Geometry: final body of the model. Coordinates: model frame, mm. Give positions to 0.01 mm unless a question says otherwise; leave off trailing zeros. Write each loop counter-clockwise with the first axis right and the second up, starting at its lowest first coordinate (ties: lowest second). Pieces come first, ordered by that corner, then holes. Notation, with made-up numbers: (59.25, 35) -> (75.25, 35) arc R10 cw to (75.25, 48) -> close; hole circle Ø2 at (84, 57). An arc over 180 degrees is marked (long way). Answer as a JSON object with one key per item and string values. Group by question number.
(1) Section query D-D on x = -14.5. Output: boundary loops of the cut face in (y, z), plus the area to 3 significant figures.
(2) Section query C-C on y = 34. Output: boundary loops of the cut face in (x, z).
(3) Section query B-B on z = 2.1. State how many separate pieces and enclosed holes the cut face has, plus the area to 3 significant figures.
(4) Material intervals for probe 1 along X at (y, z) = (50.5, 0.8); probe 2 along X at (y, z) = (43, 0.5); probe 3 along Y at (x, z) = (-8.5, 0.2), sorted ascending.
(5) Draft query along Y for faces 1 (the face through (8.02, 59.215, 1.479)), 2 (the face through (-50.516, 22.142, 1.479)), 3 (the face through (-26.851, 41.377, 1.521)), 4 (the face through (8.1, 50.194, 1.479)). Return one class per face: +Y half, -Y half, draft (parallel to the pull), parting line (faces both ways), or undercut.
(6) Contact query for a flat-ended pin moving along its axis: pin 1 Ø4 at (x, y) = (-42.89, 18.39) entering from -Z. Output: stop coordinate, or through.
(7) Section query A-A on x = 6.5. Output: boundary loops of the cut face in (y, z).
Autodesk Inventor part; units mm, degrees
ref_plane "YZ Plane" through (0, 0, 0) normal (1, 0, 0) x (0, 1, 0)
ref_plane "XZ Plane" through (0, 0, 0) normal (0, 1, 0) x (-1, 0, 0)
ref_plane "XY Plane" through (0, 0, 0) normal (0, 0, 1) x (1, 0, 0)
sketch "スケッチ1" plane through (0, 0, 0) normal (0, 0, 1) x (1, 0, 0)
  circle A0 centre (0, 0) radius 20.55 construction
  circle A1 centre (-21.6908, -16.4118) radius 19.1 construction
  circle A2 centre (25.3202, -9.9362) radius 19.1 construction
  circle A3 centre (-50.601, 30.8143) radius 1.5
  circle A4 centre (5.9362, 53.5882) radius 1.5
  circle A5 centre (27.3908, 10.6821) radius 1.5
  circle A6 centre (-42.8914, 18.3887) radius 1.5
  circle A7 centre (-21.6908, -16.4118) radius 4.025
  circle A8 centre (25.3202, -9.9362) radius 4.025
  circle A9 centre (0, 0) radius 4
  line L0 (-17.8785, -18.8026) -> (-30.4168, -38.7963) construction
  arc A10 (-17.8785, -18.8026) -> (-19.2493, -12.6317) centre (-21.6908, -16.4118) ccw construction
  line L1 (-19.2493, -12.6317) -> (-39.0737, 0.1727) construction
  line L2 (37.1409, -30.8522) -> (21.8866, -12.8448) construction
  arc A11 (22.3659, -6.5417) -> (21.8866, -12.8448) centre (25.3202, -9.9362) ccw construction
  line L3 (22.3659, -6.5417) -> (40.1678, 8.9519) construction
  line L4 (-21.6908, -16.4118) -> (-99.9742, 13.5882) construction
  line L5 (-105.5257, -16.4118) -> (-21.6908, -16.4118) construction
  line L6 (-21.6908, -16.4118) -> (-101.7113, -41.4118) construction
  line L7 (25.3202, -9.9362) -> (102.5386, -46.4118) construction
  line L8 (110.4743, -16.4118) -> (25.3202, -9.9362) construction
  line L9 (25.3202, -9.9362) -> (108.6869, 8.5882) construction
  line L10 (-18.0583, -13.7557) -> (-31.9879, 5.2949) construction
  line L11 (-17.339, -17.5569) -> (-24.5367, -44.9106) construction
  line L12 (21.5077, -7.5456) -> (34.045, 12.4488) construction
  line L13 (21.0739, -11.4259) -> (31.6059, -41.446) construction
  arc A12 (-24.6176, -40.3201) -> (-19.5065, -44.4166) centre (-20.132, -39.9603) ccw
  circle A13 centre (-20.132, -39.9603) radius 3 construction
  arc A14 (-38.9879, 7.9907) -> (-39.3359, 8.5262) centre (-35.3982, 10.7044) ccw construction
  circle A15 centre (-35.3982, 10.7044) radius 3 construction
  arc A16 (-31.9879, 5.2949) -> (-33.8465, 6.7744) centre (-35.6204, 2.6388) ccw construction
  circle A17 centre (-41.5152, -3.6073) radius 1.5
  line L14 (-33.8465, 6.7744) -> (-56.066, 16.3055) construction
  line L15 (-41.3386, 0.8892) -> (-72.6317, 2.1181) construction
  circle A18 centre (-42.8914, 18.3887) radius 3 construction
  circle A19 centre (-35.3982, 10.7044) radius 1.5
  circle A20 centre (36.7736, 17.5344) radius 1.5
  arc A21 (40.7942, 15.5132) -> (40.1934, 20.4593) centre (36.7736, 17.5344) ccw
  circle A22 centre (25.6508, -33.5339) radius 1.5
  arc A23 (26.2763, -37.9902) -> (30.1508, -33.5178) centre (25.6508, -33.5339) ccw
  circle A24 centre (36.7736, 17.5344) radius 3 construction
  circle A25 centre (25.6508, -33.5339) radius 3 construction
  arc A26 (36.6836, 14.4025) -> (34.045, 12.4488) centre (37.8575, 10.0583) ccw construction
  line L16 (36.6836, 14.4025) -> (64.1968, 21.8369) construction
  line L17 (43.2599, 10.0553) -> (82.9273, 8.8396) construction
  circle A27 centre (27.3908, 10.6821) radius 3 construction
  circle A28 centre (-21.6908, -16.4118) radius 7.025 construction
  circle A29 centre (25.3202, -9.9362) radius 7.025 construction
  arc A30 (40.8593, 15.6483) -> (30.1508, -33.5178) centre (146.4685, -33.1029) ccw
  arc A31 (-24.6176, -40.3201) -> (-39.1827, 8.2484) centre (-145.1158, -49.988) ccw
  arc A32 (-52.2824, 34.9884) -> (-54.1907, 28.1005) centre (-50.601, 30.8143) ccw
  arc A33 (9.356, 56.5132) -> (4.2549, 57.7623) centre (5.9362, 53.5882) ccw
  line L18 (-39.1827, 8.2484) -> (-54.1907, 28.1005)
  line L19 (-52.2824, 34.9884) -> (4.2549, 57.7623)
  line L20 (9.356, 56.5132) -> (40.1934, 20.4593)
  line L21 (-19.5065, -44.4166) -> (26.2763, -37.9902)
  circle A34 centre (-20.132, -39.9603) radius 1.5
  line L22 (-23.8868, -42.4405) -> (-17.339, -17.5569)
  arc A35 (-17.339, -17.5569) -> (-18.0583, -13.7557) centre (-21.6908, -16.4118) ccw
  line L23 (-18.0583, -13.7557) -> (-31.9879, 5.2949)
  arc A36 (-31.9879, 5.2949) -> (-33.8465, 6.7744) centre (-35.6204, 2.6388) ccw
  line L24 (-33.8465, 6.7744) -> (-40.0946, 9.4545)
  line L25 (40.7974, 15.5141) -> (36.6836, 14.4025)
  arc A37 (36.6836, 14.4025) -> (34.045, 12.4488) centre (37.8575, 10.0583) ccw
  line L26 (34.045, 12.4488) -> (21.5077, -7.5456)
  arc A38 (21.5077, -7.5456) -> (21.0739, -11.4259) centre (25.3202, -9.9362) ccw
  line L27 (21.0739, -11.4259) -> (29.592, -35.7057)
  dimension "d0" = 8.05
  dimension "d1" = 8.05
  dimension "d2" = 8
  dimension "d3" = 20.968
  dimension "d4" = 20.968
  dimension "d5" = 17.35
  dimension "d6" = 17.35
  dimension "d7" = 16.877
  dimension "d8" = 16.877
  dimension "d9" = 20.936
  dimension "d10" = 20.936
  dimension "d11" = 9
  dimension "d12" = 6
  dimension "d13" = 9
  dimension "d14" = 6
  dimension "d15" = 9
  dimension "d16" = 20.968
  dimension "d17" = 20.968
  dimension "d18" = 6
  dimension "d19" = 3
  dimension "d20" = 3
  dimension "d21" = 9
  dimension "d22" = 3
  dimension "d23" = 9
  dimension "d24" = 6
  dimension "d25" = 6
  dimension "d26" = 9
  dimension "d27" = 16.877
  dimension "d28" = 3
  dimension "d29" = 3
  dimension "d30" = 9
  dimension "d31" = 9
  dimension "d32" = 3
sketch "スケッチ2" plane through (0, 0, 0) normal (0, 0, 1) x (1, 0, 0)
  circle A0 centre (-50.601, 30.8143) radius 1.5
  circle A1 centre (-42.8914, 18.3887) radius 1.5
  circle A2 centre (5.9362, 53.5882) radius 1.5
  circle A3 centre (27.3908, 10.6821) radius 1.5
  arc A4 (-52.3846, 34.9457) -> (-54.4248, 28.4418) centre (-50.601, 30.8143) ccw
  arc A5 (-46.7151, 16.0162) -> (-43.3819, 13.9155) centre (-42.8914, 18.3887) ccw
  arc A6 (11.384, 56.1025) -> (3.5581, 59.0968) centre (5.9362, 53.5882) ccw
  arc A7 (26.9003, 6.2089) -> (31.4766, 12.5678) centre (27.3908, 10.6821) ccw
  line L0 (-46.7151, 16.0162) -> (-54.4248, 28.4418)
  line L1 (-52.3846, 34.9457) -> (3.5581, 59.0968)
  line L2 (11.384, 56.1025) -> (31.4766, 12.5678)
  line L3 (26.9003, 6.2089) -> (-43.3819, 13.9155)
  circle A8 centre (5.9362, 53.5882) radius 4.025
  point P0 (0, 0)
  dimension "d33" = 3
  dimension "d34" = 3
  dimension "d35" = 4.5
  dimension "d36" = 3
  dimension "d39" = 8.05
extrude "押し出し1" add sketch "スケッチ2" along normal blind 3 contours L1 A6 L2 A7 L3 A5 L0 A4
sketch "スケッチ3" plane through (0, 0, 3) normal (0, 0, 1) x (1, 0, 0)
  circle A0 centre (5.9362, 53.5882) radius 4.025
  circle A1 centre (27.3908, 10.6821) radius 1.5
  circle A2 centre (-42.8914, 18.3887) radius 1.5
  circle A3 centre (-50.601, 30.8143) radius 1.5
  line L0 (-54.4248, 28.4418) -> (-46.7151, 16.0162)
  arc A4 (-46.7151, 16.0162) -> (-43.3819, 13.9155) centre (-42.8914, 18.3887) ccw
  line L1 (-43.3819, 13.9155) -> (26.9003, 6.2089)
  arc A5 (26.9003, 6.2089) -> (31.4766, 12.5678) centre (27.3908, 10.6821) ccw
  line L2 (31.4766, 12.5678) -> (11.384, 56.1025)
  arc A6 (11.384, 56.1025) -> (3.5581, 59.0968) centre (5.9362, 53.5882) ccw
  line L3 (3.5581, 59.0968) -> (-52.3846, 34.9457)
  arc A7 (-52.3846, 34.9457) -> (-54.4248, 28.4418) centre (-50.601, 30.8143) ccw
  circle A8 centre (5.9362, 53.5882) radius 6
  circle A9 centre (-26.5254, 42.8418) radius 1.5
  circle A10 centre (-4.491, 52.3543) radius 1.5
  circle A11 centre (-4.491, 52.3543) radius 4.5 construction
  point P0 (0, 0)
  dimension "d40" = 12
  dimension "d41" = 3
  dimension "d42" = 3
  dimension "d43" = 3
  dimension "d44" = 3
  dimension "d45" = 24
  dimension "d46" = 9
extrude "押し出し2" cut sketch "スケッチ3" against normal blind 10 contours A9 | A10
equation "\"d4\" = d3"
equation "\"d6\" = d5"
equation "\"d8\" = d7"
equation "\"d10\" = d9"
equation "\"d16\" = d3"
equation "\"d17\" = d3"
equation "\"d27\" = d7"
properties part number "中間外フレーム2" material "ポリカーボネート、クリア"
Answer list:
{
 "1": {"outline": "(10.75, 0) -> (51.3, 0) -> (51.3, 3) -> (10.75, 3) -> close", "area": "122 mm2"},
 "2": {"outline": "(-53.78, 0) -> (21.58, 0) -> (21.58, 3) -> (-53.78, 3) -> close"},
 "3": {"separate pieces": "1", "enclosed holes": "6", "area": "2,810 mm2"},
 "4": {"probe 1": "-16.36 to 3.35, 8.52 to 13.97", "probe 2": "-33.73 to -28.02, -25.03 to 17.43", "probe 3": "10.09 to 53.89"},
 "5": {"face 1": "+Y half", "face 2": "-Y half", "face 3": "undercut", "face 4": "undercut"},
 "6": {"pin 1": "z = 0"},
 "7": {"outline": "(8.45, 0) -> (49.6, 0) -> (49.6, 3) -> (8.45, 3) -> close; (57.57, 0) -> (59.56, 0) -> (59.56, 3) -> (57.57, 3) -> close"}
}
